For this review, take the finished solid that the model builds, in its own axes (mm). A direction names the side the tool comes from. Give positions to 0.01 mm unless a question says otherwise; leave off trailing zeros. Order: outer loops, then holes, each group sorted by start corner. A loop starts at its lowest first (then second) coordinate and runs counter-clockwise, first axis right, second up. Notation, with made-up numbers: (-2, 73) -> (28, 73) arc R12 cw to (28, 95) -> close; hole circle Ø1 at (69, 84). An arc over 180 degrees is marked (long way). Return JSON: item names as keys, results as strings. Group by question number.
1) To check wall thickness, follow line 1 along X through (y, z) = (-8.5, -6.75); line 2 along X through (y, z) = (-6.5, -0.25); line 3 along Y through (x, z) = (-1.5, -6) (3 decimals). State the ranges of each line that lie inside material, in increasing order.
2) The part is to be moulded in two halves that separate along X. For faces 5 (the face through (56.134, -6, -9)), 6 (the face through (5.842, -2, 14)), 7 (the face through (10.16, 6, -9)), 8 (the face through (-5.622, -1.654, 9.624)), say which applies: released by +X, released by -X, zero draft, split by the parting line, or undercut.
3) Add section A-A (z = 0). Give the boundary of the cut face in (x, y) (3 decimals).
4) Add section B-B (y = 0). Give the boundary of the cut face in (x, z) (3 decimals).
5) Add section D-D (y = 9). Give the boundary of the cut face in (x, z), then the cut area to 3 significant figures.
6) Insertion check: P1, Ø12, axis at y = -1, z = -8, coming from the -X side; P2, Ø1.3, axis at y = -3.5, z = 14, coming from the +X side; P3, Ø3, axis at x = 25, y = -1, coming from the +Z side. Each pin has a flat end and moves straight along its axis. Give the tip position at first contact, or say it passes through.
7) For faces 1 (the face through (61, -6.35, 12)), 2 (the face through (0, 6, -3)), 3 (the face through (32.825, 2.174, -9.925)), 4 (the face through (33, -2, 10.16)), list the 3-axis set-ups (+Z, -Z, +X, -X, +Y, -Y) from which the entire face can be reached by the end or side of a thin tool; tool diameter is ignored.
8) Add section C-C (x = 39). Give the boundary of the cut face in (y, z) (3 decimals).
from build123d import *

# Parameters (mm, degrees)
F0_W     = 5.842
F0_H     = 12.7
F0_R     = 3.175
F2_DEPTH = 6.35
F3_DEPTH = 6.35
F4_DEPTH = 3.175
F5_DEPTH = 3.175


# Not quite as in the source:
# - the program builds the solid bodies; features that only make, move or delete a surface that nothing else refers to are left out


with BuildPart() as f1:
    # F0 (on Front) → F1 (revolve)
    with BuildSketch(Plane.XZ):
        Polygon((5.842, 12.7), (5.842, 0), (66.294, 0), (66.294, 12.7), (56.134, 12.7), (56.134, 10.16), (10.16, 10.16), (10.16, 12.7), align=None)
        with Locations((2.921, 6.35)):
            Rectangle(F0_W, F0_H)
    revolve(axis=Axis((33.147, 0, 0), (-1, 0, 0)))

    # F0 (on Front) → F2 (join)
    with BuildSketch(Plane.XZ):
        Polygon((5.842, 12.7), (5.842, 0), (66.294, 0), (66.294, 12.7), (56.134, 12.7), (56.134, 10.16), (10.16, 10.16), (10.16, 12.7), align=None)
        with BuildLine():
            ThreePointArc((-8.1826630726, -5.5069827884), (-3.1957909266, -4.5493385486), (-0.9398, 0))
            ThreePointArc((-0.9398, 0), (-4.5919612295, 5.3297205562), (-10.8806298187, 3.8475430269))
            ThreePointArc((-10.8806298187, 3.8475430269), (-12.1459778134, -1.5837270034), (-8.1826630726, -5.5069827884))
        make_face()
        with Locations((-6.6548, 0)):
            Circle(F0_R, mode=Mode.SUBTRACT)
        with Locations((2.921, 6.35)):
            Rectangle(F0_W, F0_H)
        with BuildLine():
            Line((5.842, 0), (0, 0))
            Line((0, 0), (-0.9398, 0))
            ThreePointArc((-0.9398, 0), (-3.1957909266, -4.5493385486), (-8.1826630726, -5.5069827884))
            Line((-8.1826630726, -5.5069827884), (5.842, -9.398))
            Line((5.842, -9.398), (5.842, 0))
        make_face()
        with Locations((-6.6548, 0)):
            Circle(F0_R)
    extrude(amount=F2_DEPTH)

    # F0 (on Front) → F3 (join)
    with BuildSketch(Plane.XZ):
        with BuildLine():
            Line((-0.9398, 0), (0, 0))
            Line((0, 0), (0, 12.7))
            Line((0, 12.7), (5.842, 12.7))
            Line((5.842, 12.7), (5.842, 15.24))
            Line((5.842, 15.24), (-0.508, 15.24))
            Line((-0.508, 15.24), (-10.8806298187, 3.8475430269))
            ThreePointArc((-10.8806298187, 3.8475430269), (-4.5919612295, 5.3297205562), (-0.9398, 0))
        make_face()
    extrude(amount=F3_DEPTH)

    # F0 (on Front) → F4 (join, symmetric)
    with BuildSketch(Plane.XZ):
        with BuildLine():
            Line((-0.9398, 0), (0, 0))
            Line((0, 0), (0, 12.7))
            Line((0, 12.7), (5.842, 12.7))
            Line((5.842, 12.7), (5.842, 15.24))
            Line((5.842, 15.24), (-0.508, 15.24))
            Line((-0.508, 15.24), (-10.8806298187, 3.8475430269))
            ThreePointArc((-10.8806298187, 3.8475430269), (-4.5919612295, 5.3297205562), (-0.9398, 0))
        make_face()
        with Locations((2.921, 6.35)):
            Rectangle(F0_W, F0_H)
        with BuildLine():
            Line((5.842, 0), (0, 0))
            Line((0, 0), (-0.9398, 0))
            ThreePointArc((-0.9398, 0), (-3.1957909266, -4.5493385486), (-8.1826630726, -5.5069827884))
            Line((-8.1826630726, -5.5069827884), (5.842, -9.398))
            Line((5.842, -9.398), (5.842, 0))
        make_face()
        Polygon((5.842, 12.7), (5.842, 0), (66.294, 0), (66.294, 12.7), (56.134, 12.7), (56.134, 10.16), (10.16, 10.16), (10.16, 12.7), align=None)
        with BuildLine():
            ThreePointArc((-8.1826630726, -5.5069827884), (-3.1957909266, -4.5493385486), (-0.9398, 0))
            ThreePointArc((-0.9398, 0), (-4.5919612295, 5.3297205562), (-10.8806298187, 3.8475430269))
            ThreePointArc((-10.8806298187, 3.8475430269), (-12.1459778134, -1.5837270034), (-8.1826630726, -5.5069827884))
        make_face()
        with Locations((-6.6548, 0)):
            Circle(F0_R, mode=Mode.SUBTRACT)
    extrude(amount=F4_DEPTH, both=True)

    # F0 (on Front) → F5 (join, symmetric)
    with BuildSketch(Plane.XZ):
        Polygon((5.842, 12.7), (5.842, 0), (66.294, 0), (66.294, 12.7), (56.134, 12.7), (56.134, 10.16), (10.16, 10.16), (10.16, 12.7), align=None)
        with BuildLine():
            ThreePointArc((-8.1826630726, -5.5069827884), (-3.1957909266, -4.5493385486), (-0.9398, 0))
            ThreePointArc((-0.9398, 0), (-4.5919612295, 5.3297205562), (-10.8806298187, 3.8475430269))
            ThreePointArc((-10.8806298187, 3.8475430269), (-12.1459778134, -1.5837270034), (-8.1826630726, -5.5069827884))
        make_face()
        with Locations((-6.6548, 0)):
            Circle(F0_R, mode=Mode.SUBTRACT)
        with BuildLine():
            Line((-0.9398, 0), (0, 0))
            Line((0, 0), (0, 12.7))
            Line((0, 12.7), (5.842, 12.7))
            Line((5.842, 12.7), (5.842, 15.24))
            Line((5.842, 15.24), (-0.508, 15.24))
            Line((-0.508, 15.24), (-10.8806298187, 3.8475430269))
            ThreePointArc((-10.8806298187, 3.8475430269), (-4.5919612295, 5.3297205562), (-0.9398, 0))
        make_face()
        with Locations((2.921, 6.35)):
            Rectangle(F0_W, F0_H)
        with BuildLine():
            Line((5.842, 0), (0, 0))
            Line((0, 0), (-0.9398, 0))
            ThreePointArc((-0.9398, 0), (-3.1957909266, -4.5493385486), (-8.1826630726, -5.5069827884))
            Line((-8.1826630726, -5.5069827884), (5.842, -9.398))
            Line((5.842, -9.398), (5.842, 0))
        make_face()
        with Locations((-6.6548, 0)):
            Circle(F0_R)
    extrude(amount=F5_DEPTH, both=True)


solid = f1.part
Evaluation:
{
 "1": {"line 1": "0 to 10.16, 56.13 to 66.29", "line 2": "0 to 66.29", "line 3": "-6.35 to 3.175"},
 "2": {"face 5": "undercut", "face 6": "released by +X", "face 7": "undercut", "face 8": "released by -X"},
 "3": {"outline": "(-12.37, -6.35) -> (0, -6.35) -> (0, -12.7) -> (10.16, -12.7) -> (10.16, -10.16) -> (56.134, -10.16) -> (56.134, -12.7) -> (66.294, -12.7) -> (66.294, 12.7) -> (56.134, 12.7) -> (56.134, 10.16) -> (10.16, 10.16) -> (10.16, 12.7) -> (0, 12.7) -> (0, 3.175) -> (-12.37, 3.175) -> close"},
 "4": {"outline": "(-10.881, 3.848) arc R5.715 ccw to (-8.183, -5.507) -> (0, -7.777) -> (0, -12.7) -> (10.16, -12.7) -> (10.16, -10.16) -> (56.134, -10.16) -> (56.134, -12.7) -> (66.294, -12.7) -> (66.294, 12.7) -> (56.134, 12.7) -> (56.134, 10.16) -> (10.16, 10.16) -> (10.16, 12.7) -> (5.842, 12.7) -> (5.842, 15.24) -> (-0.508, 15.24) -> close"},
 "5": {"outline": "(0, -8.96) -> (10.16, -8.96) -> (10.16, -4.71) -> (56.13, -4.71) -> (56.13, -8.96) -> (66.29, -8.96) -> (66.29, 8.96) -> (56.13, 8.96) -> (56.13, 4.71) -> (10.16, 4.71) -> (10.16, 8.96) -> (0, 8.96) -> close", "area": "798 mm^2"},
 "6": {"P1": "x = -12.01", "P2": "x = 5.84", "P3": "z = 10.16"},
 "7": {"face 1": "+Z, +X, -X, -Y", "face 2": "-Z, -X", "face 3": "none", "face 4": "+Z, +Y, -Y"},
 "8": {"outline": "(-6.35, 7.931) arc R10.16 ccw (long way) to (3.175, 9.651) -> (3.175, 10.16) -> (-6.35, 10.16) -> close"}
}
